Can you work these out from the drawing? Everything is in mm from the part's minimum corner. A direction names the side the tool comes from. Coordinates: 2 decimals unless noted, no trailing zeros. Loops run counter-clockwise (first coordinate to the right, second up) from the corner with the lowest first, then second, coordinate; pieces in that order, holes last.
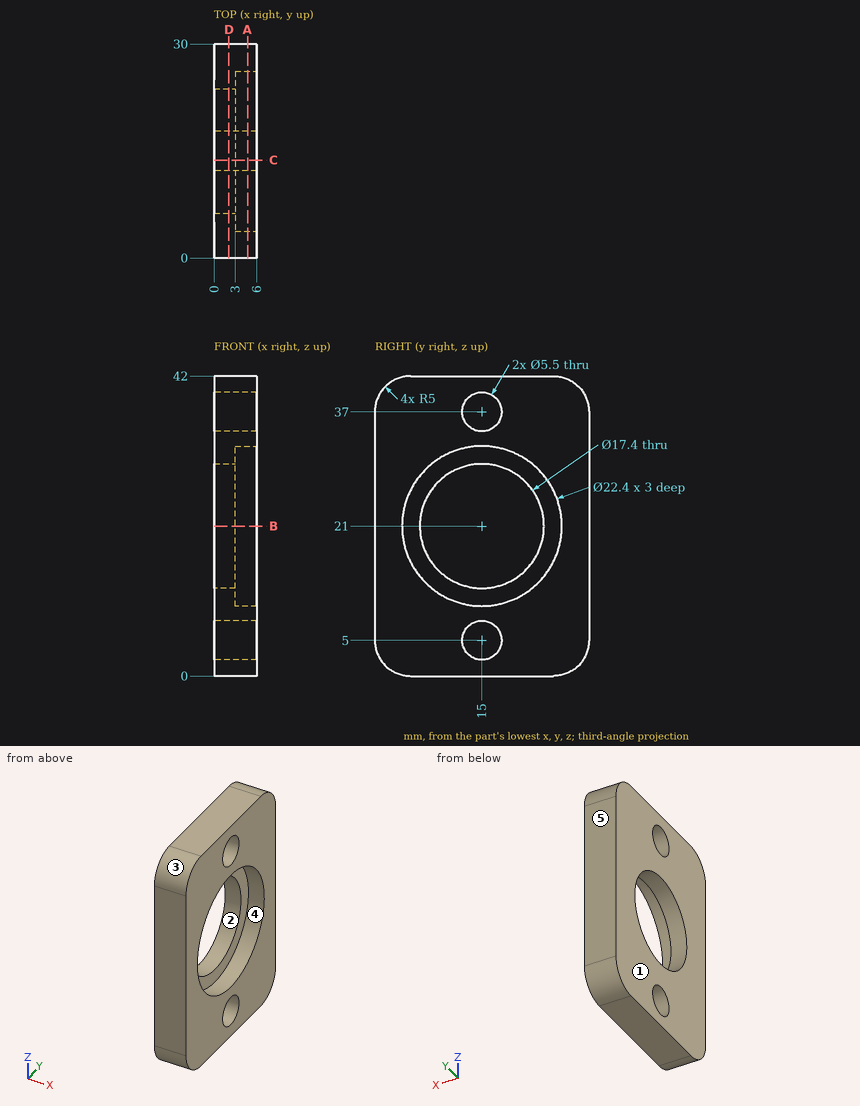
(1) Imagine slicing it at B-B, the plane z = 21. Write out the boundary of the cut face in (x, y), and give its area (3 significant figures).
Answers:
outline: (0, 0) - (6, 0) - (6, 3.8) - (3, 3.8) - (3, 6.3) - (0, 6.3) - close; (0, 23.7) - (3, 23.7) - (3, 26.2) - (6, 26.2) - (6, 30) - (0, 30) - close
area: 60.6 mm2
(2) Imagine slicing it at A-A, the plane x = 4.7. Write out the boundary of the cut face in (y, z), and give its area (3 significant figures).
Answers:
outline: (0, 5) arc R5 ccw to (5, 0) - (25, 0) arc R5 ccw to (30, 5) - (30, 37) arc R5 ccw to (25, 42) - (5, 42) arc R5 ccw to (0, 37) - close; hole circle Ø22.4 at (15, 21); hole circle Ø5.5 at (15, 5); hole circle Ø5.5 at (15, 37)
area: 797 mm2
(3) Imagine slicing it at D-D, the plane x = 2.1. Write out the boundary of the cut face in (y, z).
Answers:
outline: (0, 5) arc R5 ccw to (5, 0) - (25, 0) arc R5 ccw to (30, 5) - (30, 37) arc R5 ccw to (25, 42) - (5, 42) arc R5 ccw to (0, 37) - close; hole circle Ø17.4 at (15, 21); hole circle Ø5.5 at (15, 5); hole circle Ø5.5 at (15, 37)
(4) For pin 1 (6 mm diameter, centred on y = 7, z = 15, fed in from +X); pin 2 (11 mm diameter, centred on y = 19, z = 24.5, fed in from +X), each with a flat end and sliding along its axis, tell me the tip position at first contact or that it passes through.
Answers:
pin 1: stops at x = 6
pin 2: stops at x = 3
(5) I need wall thicknesses on probe 1 along Y at (x, z) = (4.65, 37); probe 2 along Y at (x, z) = (0.9, 21); probe 3 along Z at (x, y) = (4.15, 21.5). Which ranges of each line are inside material? Lowest first, please.
Answers:
probe 1: y = 0 to 12.25, 17.75 to 30
probe 2: y = 0 to 6.3, 23.7 to 30
probe 3: z = 0 to 11.88, 30.12 to 42
(6) Imagine slicing it at C-C, the plane y = 13.75. Write out the boundary of the cut face in (x, z).
Answers:
outline: (0, 0) - (6, 0) - (6, 2.55) - (0, 2.55) - close; (0, 7.45) - (6, 7.45) - (6, 9.87) - (3, 9.87) - (3, 12.39) - (0, 12.39) - close; (0, 29.61) - (3, 29.61) - (3, 32.13) - (6, 32.13) - (6, 34.55) - (0, 34.55) - close; (0, 39.45) - (6, 39.45) - (6, 42) - (0, 42) - close
(7) We'd pull the mould along Z, two halves only. Please class the marked faces 1, 2 and 3: +Z half, -Z half, draft (parallel to the pull), parting line (faces both ways), or undercut.
Answers:
face 1: draft
face 2: undercut
face 3: +Z half
(8) Which directions (+Z, -Z, +X, -X, +Y, -Y) give clear straight access to the entire face, cutting with the end or side of a thin tool? Please do the marked faces 4 and 5.
Answers:
face 4: +X
face 5: +Z, -Z, +X, -X, +Y
